Geometry check sheet. Reference: the model listing, model coordinates, mm. Face numbers are marked on the shaded views. A direction names the side the tool comes from. Give positions to 0.01 mm unless a question says otherwise; leave off trailing zeros. Loops run counter-clockwise (first coordinate to the right, second up) from the corner with the lowest first, then second, coordinate; pieces in that order, holes last. Notation, with made-up numbers: (-6.75, 82) - (-2.75, 82) arc R20 cw to (-2.75, 87) - close; hole circle Ø4 at (20.25, 75). An arc over 180 degrees is marked (long way). One line per question, with ' | ' between items. Start each with the question number.
from build123d import *

# Parameters (mm, degrees)
EXTRUDE_1_DEPTH     = 14
CUT_EXTRUDE_START   = -26
SKETCH_2_R          = 3.5
CUT_EXTRUDE_1_DEPTH = 26
SKETCH_3_R          = 2.75
CUT_EXTRUDE_2_DEPTH = 14


with BuildPart() as part:
    # 草图1 → 凸台-拉伸1 (new body)
    with BuildSketch(Plane.XY):
        with BuildLine():
            Line((4.326086957, 24.059506973), (-7.173913043, 24.059506973))
            Line((-7.173913043, 24.059506973), (-7.173913043, -14.940493027))
            Line((-7.173913043, -14.940493027), (-19.173913043, -14.940493027))
            Line((-19.173913043, -14.940493027), (-19.173913043, -20.940493027))
            Line((-19.173913043, -20.940493027), (30.826086957, -20.940493027))
            Line((30.826086957, -20.940493027), (30.826086957, -14.940493027))
            Line((30.826086957, -14.940493027), (18.826086957, -14.940493027))
            Line((18.826086957, -14.940493027), (18.826086957, 24.059506973))
            Line((18.826086957, 24.059506973), (7.326086957, 24.059506973))
            Line((7.326086957, 24.059506973), (7.326086957, 6.917623795))
            ThreePointArc((7.326086957, 6.917623795), (11.990500959, 4.158526486), (13.826086957, -0.940493027))
            ThreePointArc((13.826086957, -0.940493027), (0.727067443, -7.10490703), (4.326086957, 6.917623795))
            Line((4.326086957, 6.917623795), (4.326086957, 24.059506973))
        make_face()
    extrude(amount=EXTRUDE_1_DEPTH)

    # 草图2 → 切除-拉伸1 (cut)
    with BuildSketch(Plane(origin=(18.826086957, 0, 0), x_dir=(0, 0, -1), z_dir=(1, 0, 0)).offset(CUT_EXTRUDE_START)):
        with Locations(Location((-7, 12.059506973, 0), (0, 0, 90))):
            Circle(SKETCH_2_R)
    extrude(amount=CUT_EXTRUDE_1_DEPTH, mode=Mode.SUBTRACT)

    # 草图3 → 切除-拉伸2 (cut)
    with BuildSketch(Plane(origin=(0, -20.940493027, 0), x_dir=(-1, 0, 0), z_dir=(0, -1, 0))):
        with Locations(Location((14.173913043, -7, 0), (0, 0, 180))):
            Circle(SKETCH_3_R)
        with Locations(Location((-25.826086957, -7, 0), (0, 0, 90))):
            Circle(SKETCH_3_R)
    extrude(amount=-CUT_EXTRUDE_2_DEPTH, mode=Mode.SUBTRACT)


solid = part.part
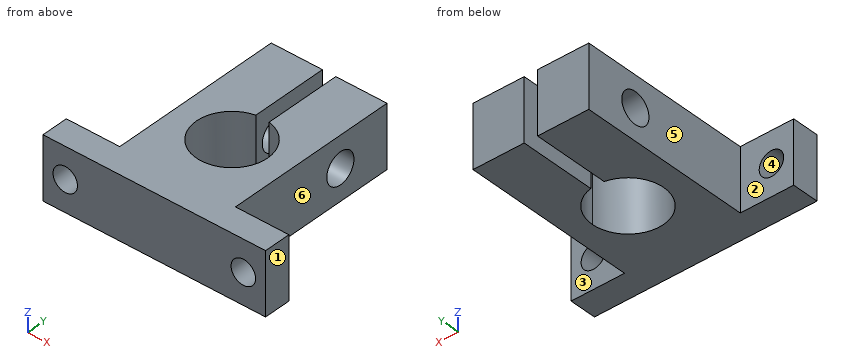
(1) Mould release check, pull along X, two halves, no side actions. Record for the marked faces 3, 4, 5 and 6: pulls with the +X half, pulls with the -X half, needs draft (parallel to the pull), parting line crosses it, or undercut.
(2) Section check C-C, the plane x = 26.5. Record the boundary of the cut face in (y, z), and give its area (3 significant figures).
(3) Depth check by flat-ended pin: pin 1 Ø1.5 at (x, y) = (4, -8) entering from -Z; pin 2 Ø7 at (y, z) = (17, 7) entering from -X; pin 3 Ø3.5 at (x, z) = (23.5, 5) entering from +Y. Enter the tip coordinate at first touch or a pass-through.
(4) Material ranges on line 1 (X direction, y = -0.5, z = 9.5); line 2 (Y direction, x = 10, z = 7); line 3 (Y direction, x = 1, z = 8), recorded low to high.
(5) Tool access check on the marked faces 1 and 2. Record the directions out of +Z, -Z, +X, -X, +Y, -Y that give a thin tool (end or side, any length) a straight path to the whole face; none if there is none.
(6) Section check D-D, the plane z = 1.5. Record the boundary of the cut face in (x, y).
(7) Section check A-A, the plane z = 7. Record the boundary of the cut face in (x, y), and give its area (3 significant figures).
(8) Section check B-B, the plane y = 13. Record the boundary of the cut face in (x, z), and give its area (3 significant figures).
Numbers:
1) face 3: needs draft | face 4: undercut | face 5: pulls with the -X half | face 6: pulls with the +X half
2) outline: (-20.94, 0) - (-14.94, 0) - (-14.94, 4.33) - (-20.94, 4.33) - close; (-20.94, 9.67) - (-14.94, 9.67) - (-14.94, 14) - (-20.94, 14) - close | area: 52.0 mm^2
3) pin 1: z = 0 | pin 2: x = -7.17 | pin 3: y = -14.94
4) line 1: -7.17 to -2.16, 13.81 to 18.83 | line 2: -20.94 to -7.77, 5.88 to 8.56, 15.56 to 24.06 | line 3: -20.94 to -7.32, 5.44 to 8.71, 15.41 to 24.06
5) face 1: +Z, -Z, +X, +Y, -Y | face 2: +Z, -Z, -X, +Y
6) outline: (-19.17, -20.94) - (30.83, -20.94) - (30.83, -14.94) - (18.83, -14.94) - (18.83, 24.06) - (7.33, 24.06) - (7.33, 6.92) arc R8 cw (long way) to (4.33, 6.92) - (4.33, 24.06) - (-7.17, 24.06) - (-7.17, -14.94) - (-19.17, -14.94) - close
7) outline: (-19.17, -20.94) - (-16.92, -20.94) - (-16.92, -14.94) - (-19.17, -14.94) - close; (-11.42, -20.94) - (23.08, -20.94) - (23.08, -14.94) - (18.83, -14.94) - (18.83, 8.56) - (7.33, 8.56) - (7.33, 6.92) arc R8 cw (long way) to (4.33, 6.92) - (4.33, 8.56) - (-7.17, 8.56) - (-7.17, -14.94) - (-11.42, -14.94) - close; (-7.17, 15.56) - (4.33, 15.56) - (4.33, 24.06) - (-7.17, 24.06) - close; (7.33, 15.56) - (18.83, 15.56) - (18.83, 24.06) - (7.33, 24.06) - close; (28.58, -20.94) - (30.83, -20.94) - (30.83, -14.94) - (28.58, -14.94) - close | area: 835 mm^2
8) outline: (-7.17, 0) - (4.33, 0) - (4.33, 3.63) - (-7.17, 3.63) - close; (-7.17, 10.37) - (4.33, 10.37) - (4.33, 14) - (-7.17, 14) - close; (7.33, 0) - (18.83, 0) - (18.83, 3.63) - (7.33, 3.63) - close; (7.33, 10.37) - (18.83, 10.37) - (18.83, 14) - (7.33, 14) - close | area: 167 mm^2
